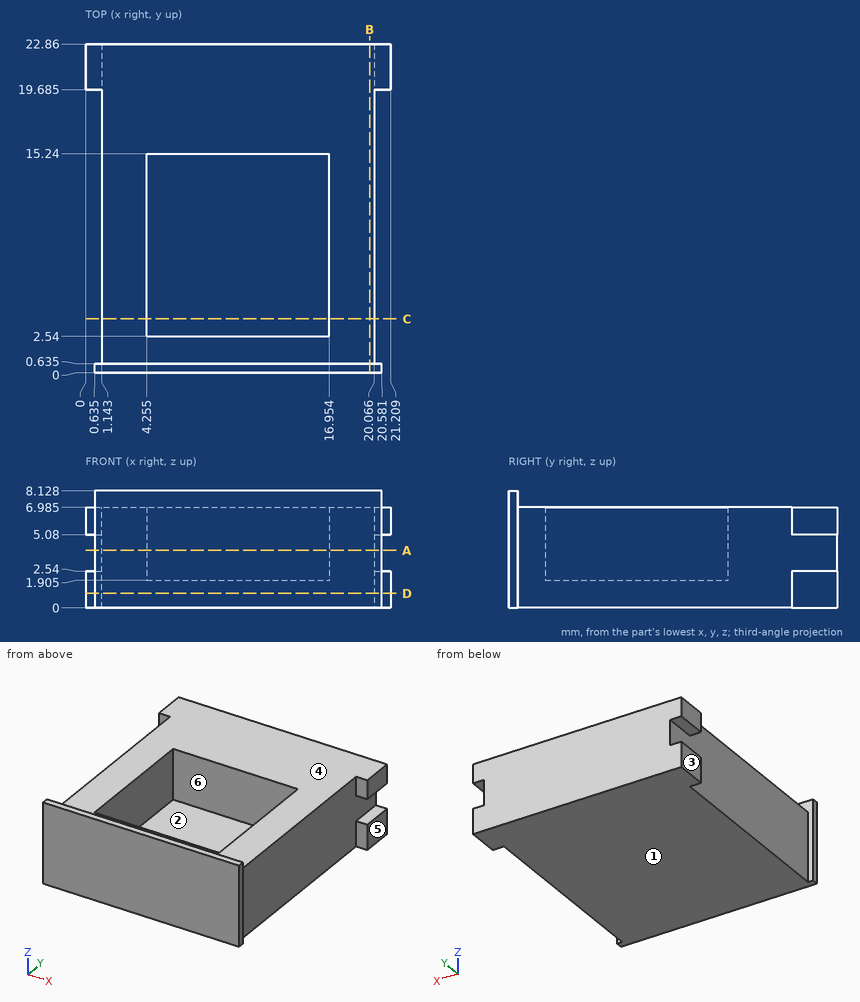
Verification items for this drawing (mm, ordinates from the low corner). A direction names the side the tool comes from. Round coordinates to 2 decimals unless told otherwise and drop trailing zeros. Write each loop counter-clockwise with the first axis right and the second up, starting at its lowest first coordinate (ties: lowest second). Pieces come first, ordered by that corner, then holes. Notation, with made-up numbers: (-21.5, 52.5) - (19.5, 52.5) arc R12 ccw to (19.5, 57.5) - close; hole circle Ø11 at (51.5, 14). An arc over 180 degrees is marked (long way). One line per item, written item: value.
1. Set-up check for the marked faces 4, 5 and 6: record each of +Z, -Z, +X, -X, +Y, -Y from which the full face is reachable in a straight line by a thin tool's end or side.
The answers:
face 4: +Z, +X, -X, +Y
face 5: +Z, -Z, +X, +Y, -Y
face 6: +Z
2. Cross-section at D-D on z = 1. Record the boundary of the cut face in (x, y) (1 decimal).
The answers:
outline: (0, 19.7) - (1.1, 19.7) - (1.1, 0.6) - (0.6, 0.6) - (0.6, 0) - (20.6, 0) - (20.6, 0.6) - (20.1, 0.6) - (20.1, 19.7) - (21.2, 19.7) - (21.2, 22.9) - (0, 22.9) - close
3. Cross-section at C-C on y = 3.75. Record the boundary of the cut face in (x, z) (1 decimal).
The answers:
outline: (1.1, 0) - (20.1, 0) - (20.1, 7) - (17, 7) - (17, 1.9) - (4.3, 1.9) - (4.3, 7) - (1.1, 7) - close
4. Scan lines: L1, parallel to Y at x = 11, z = 6; L2, parallel to X at y = 12.5, z = 2.25 (1 decimal); L3, parallel to X at y = 19, z = 6.25 (1 decimal). Record each from-to range of solid material in increasing order.
The answers:
L1: y = 0 to 2.54, 15.24 to 22.86
L2: x = 1.1 to 4.3, 17 to 20.1
L3: x = 1.1 to 20.1
5. Mould release check, pull along X, two halves, no side actions. Record for the marked faces 1, 2 and 3: released by +X, released by -X, zero draft, split by the parting line, or undercut.
The answers:
face 1: zero draft
face 2: undercut
face 3: released by -X
6. Depth check by flat-ended pin: pin 1 Ø1 at (x, y) = (10.5, 10.5) entering from +Z (1 decimal); pin 2 Ø1.5 at (y, z) = (6, 4) entering from -X; pin 3 Ø0.7 at (y, z) = (0.5, 3) entering from -X (1 decimal). Enter the tip coordinate at first touch or a pass-through.
The answers:
pin 1: stops at z = 1.9
pin 2: stops at x = 1.14
pin 3: stops at x = 0.6
7. Cross-section at B-B on x = 19.75. Record the boundary of the cut face in (y, z) (1 decimal), and give its area (3 significant figures).
The answers:
outline: (0, 0) - (22.9, 0) - (22.9, 7) - (0.6, 7) - (0.6, 8.1) - (0, 8.1) - close
area: 160 mm^2
8. Cross-section at A-A on z = 4. Record the boundary of the cut face in (x, y) (1 decimal), and give its area (3 significant figures).
The answers:
outline: (0.6, 0) - (20.6, 0) - (20.6, 0.6) - (20.1, 0.6) - (20.1, 22.9) - (1.1, 22.9) - (1.1, 0.6) - (0.6, 0.6) - close; hole (4.3, 2.5) - (17, 2.5) - (17, 15.2) - (4.3, 15.2) - close
area: 272 mm^2
